```python
from build123d import *

# Parameters (mm, degrees)
SKETCH1_W           = 98
SKETCH1_H           = 146.5
BOSS_EXTRUDE1_DEPTH = 4.2
SKETCH3_R           = 20
CUT_EXTRUDE2_DEPTH  = 10
SKETCH4_R           = 2.35
CUT_EXTRUDE3_DEPTH  = 10
CUT_EXTRUDE5_DEPTH  = 131.021293634


with BuildPart() as part:
    # Sketch1 → Boss-Extrude1 (new body)
    with BuildSketch(Plane.XY):
        with Locations((24.233695652, -34.10326087)):
            Rectangle(SKETCH1_W, SKETCH1_H)
    extrude(amount=BOSS_EXTRUDE1_DEPTH)

    # Sketch3 → Cut-Extrude2 (cut)
    with BuildSketch(Plane.XY.offset(4.2)):
        with Locations((43.233695652, 9.14673913)):
            Circle(SKETCH3_R)
    extrude(amount=-CUT_EXTRUDE2_DEPTH, mode=Mode.SUBTRACT)

    # Sketch4 → Cut-Extrude3 (cut)
    with BuildSketch(Plane.XY.offset(4.2)):
        with Locations((27.233695652, 25.14673913)):
            Circle(SKETCH4_R)
        with Locations((59.233695652, 25.14673913)):
            Circle(SKETCH4_R)
        with Locations((59.233695652, -6.85326087)):
            Circle(SKETCH4_R)
        with Locations((27.233695652, -6.85326087)):
            Circle(SKETCH4_R)
    extrude(amount=-CUT_EXTRUDE3_DEPTH, mode=Mode.SUBTRACT)

    # Sketch6 → Cut-Extrude5 (cut, through all)
    with BuildSketch(Plane.XY.offset(4.2)):
        with BuildLine():
            Line((18.233695652, -97.35326087), (30.233695652, -97.35326087))
            ThreePointArc((30.233695652, -97.35326087), (32.233695652, -99.35326087), (30.233695652, -101.35326087))
            Line((30.233695652, -101.35326087), (18.233695652, -101.35326087))
            ThreePointArc((18.233695652, -101.35326087), (16.233695652, -99.35326087), (18.233695652, -97.35326087))
        make_face()
    extrude(amount=-CUT_EXTRUDE5_DEPTH, mode=Mode.SUBTRACT)


solid = part.part
```
CAD build for the part. Positions are in the model's coordinates, mm. A direction names the side the tool comes from. Coordinates: 2 decimals unless noted, no trailing zeros. Order: outer loops, then holes, each group sorted by start corner. A loop starts at its lowest first (then second) coordinate and runs counter-clockwise, first axis right, second up. Notation, with made-up numbers: (82, -10) -> (131, -10) arc R23 cw to (131, 16) -> close; hole circle Ø5 at (85.5, 24.25). An arc over 180 degrees is marked (long way). Use one line per item in the form item = value. Start each with the question number.
1) Band-saw the part on A-A on x = 43. Give the cut face in (y, z).
2) Tool access for faces 1 (the cylindrical face through (32.233, -99.309, 2.129)), 2 (the flat face through (24, -33, 0)): list every direction of +Z, -Z, +X, -X, +Y, -Y with a clear straight run to the whole face (end or side of a thin tool).
3) Band-saw the part on B-B on y = 13. Give the cut face in (x, z).
4) Drill centre lines: L1, parallel to X at y = 9.5, z = 3.9; L2, parallel to X at y = -8, z = 2.05; L3, parallel to Y at x = 61, z = 0.9. Where is each one in solid material? Low to high. Write a range as [from, to].
5) Pull direction Y, two halves, no side cores. Call faces 3 (the cylindrical face through (29.404, -7.753, 2.129)), 4 (the flat face through (24, 39.147, 2)), 5 (the flat face through (24, -107.353, 2)), 6 (the flat face through (24, -33, 4.2)): +Y half, -Y half, draft (parallel to the pull), parting line (faces both ways), or undercut.
6) Band-saw the part on C-C on z = 3. Give the cut face in (x, y).
Entries:
q1.outline = (-107.35, 0) -> (-10.85, 0) -> (-10.85, 4.2) -> (-107.35, 4.2) -> close; (29.15, 0) -> (39.15, 0) -> (39.15, 4.2) -> (29.15, 4.2) -> close
q2.face_1 = +Z, -Z
q2.face_2 = -Z, +X, -X, +Y, -Y
q3.outline = (-24.77, 0) -> (23.61, 0) -> (23.61, 4.2) -> (-24.77, 4.2) -> close; (62.86, 0) -> (73.23, 0) -> (73.23, 4.2) -> (62.86, 4.2) -> close
q4.L1 = [-24.77, 23.24], [63.23, 73.23]
q4.L2 = [-24.77, 25.18], [29.28, 32.94], [53.53, 57.18], [61.28, 73.23]
q4.L3 = [-107.35, -8.4], [-5.3, -0.04], [18.33, 23.6], [26.7, 39.15]
q5.face_3 = undercut
q5.face_4 = +Y half
q5.face_5 = -Y half
q5.face_6 = draft
q6.outline = (-24.77, -107.35) -> (73.23, -107.35) -> (73.23, 39.15) -> (-24.77, 39.15) -> close; hole (18.23, -101.35) -> (30.23, -101.35) arc R2 ccw to (30.23, -97.35) -> (18.23, -97.35) arc R2 ccw to start; hole circle Ø40 at (43.23, 9.15); hole circle Ø4.7 at (27.23, -6.85); hole circle Ø4.7 at (27.23, 25.15); hole circle Ø4.7 at (59.23, -6.85); hole circle Ø4.7 at (59.23, 25.15)
